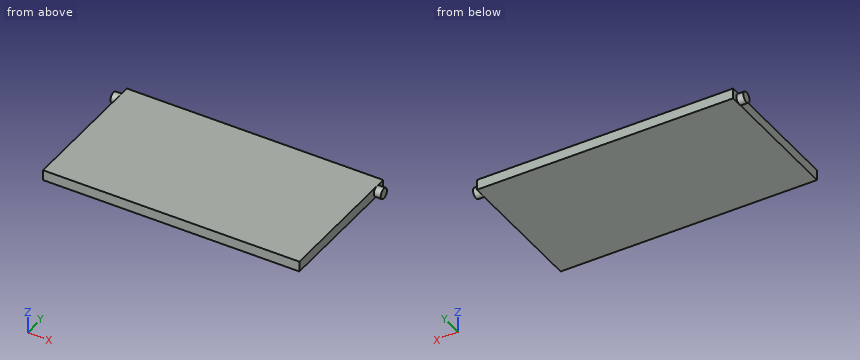
Autodesk Inventor part; units mm, degrees
ref_plane "YZ Plane" through (0, 0, 0) normal (1, 0, 0) x (0, 1, 0)
ref_plane "XZ Plane" through (0, 0, 0) normal (0, 1, 0) x (-1, 0, 0)
ref_plane "XY Plane" through (0, 0, 0) normal (0, 0, 1) x (1, 0, 0)
sketch "草图1" plane through (0, 0, 0) normal (1, 0, 0) x (0, 1, 0)
  line L0 (100, 7.5) -> (-100, 7.5)
  line L1 (-100, 7.5) -> (-100, -7.5)
  line L2 (-100, -7.5) -> (100, -7.5)
  line L3 (100, -7.5) -> (100, 7.5)
  line L4 (0, -10.5) -> (0, 10.5)
  line L5 (-140, 0) -> (140, 0)
  point P0 (0, 0)
  dimension "d0" = 15
  dimension "d1" = 200
extrude "拉伸1" add sketch "草图1" along normal mid plane 370
sketch "草图2" plane through (-185, 0, 0) normal (-1, 0, 0) x (0, 0, 1)
  line L0 (0, -148.5) -> (0, 191)
  circle A0 centre (0, 85) radius 7.5
  line L1 (7.5, 100) -> (-7.5, 100)
  point P0 (0, 0)
  dimension "d4" = 15
  dimension "d5" = 15
extrude "拉伸2" add sketch "草图2" along normal blind 10
mirror "镜像1" about plane through (0, 0, 0) normal (1, 0, 0) of "拉伸2"
properties part number "挡板"
The listing builds one solid part. Answer for the finished solid, in the listing's coordinates (mm). Give positions to 0.01 mm unless a question says otherwise; leave off trailing zeros. Order: outer loops, then holes, each group sorted by start corner. A loop starts at its lowest first (then second) coordinate and runs counter-clockwise, first axis right, second up. Notation, with made-up numbers: (60, 4) -> (119, 4) arc R27 cw to (119, 25) -> close; hole circle Ø5 at (72, 33.5). An arc over 180 degrees is marked (long way). One line per item, written item: value.
1) Flat-ended cylindrical pins translate along their axes: P1, Ø3, axis at y = 12.5, z = 0.5, coming from the +X side; P2, Ø4, axis at y = 44.5, z = 5.5, coming from the -X side. Find the tip coordinate at first contact, or state that the pin passes through.
Reported:
P1: stops at x = 185
P2: stops at x = -185
2) Find section B-B, the plane y = 42. Determine the outline of the cut face in (x, z), plus the area to 3 significant figures.
Reported:
outline: (-185, -7.5) -> (185, -7.5) -> (185, 7.5) -> (-185, 7.5) -> close
area: 5,550 mm^2
3) Find section A-A, the plane z = 0. Determine the outline of the cut face in (x, y), plus the area to 3 significant figures.
Reported:
outline: (-195, 77.5) -> (-185, 77.5) -> (-185, -100) -> (185, -100) -> (185, 77.5) -> (195, 77.5) -> (195, 92.5) -> (185, 92.5) -> (185, 100) -> (-185, 100) -> (-185, 92.5) -> (-195, 92.5) -> close
area: 74,300 mm^2
4) Find the intervals of material crossed by line 1 (X direction, y = -39, z = 0.25), in increasing order.
Reported:
line 1: x = -185 to 185
